Answer from the drawing. Dimensions are ordinates in mm from the lowest x, y and z of the part. Round coordinates to 2 decimals unless told otherwise and drop trailing zeros. Order: outer loops, then holes, each group sorted by start corner. A loop starts at its lowest first (then second) coordinate and runs counter-clockwise, first axis right, second up. Notation, with made-up numbers: M 76.5,34 L 108.5,34 A14 cw 108.5,55 Z; hole C 74.25,51.25 d4. An arc over 180 degrees is marked long. Answer as a JSON object with one key per item and string values. Group by question number.
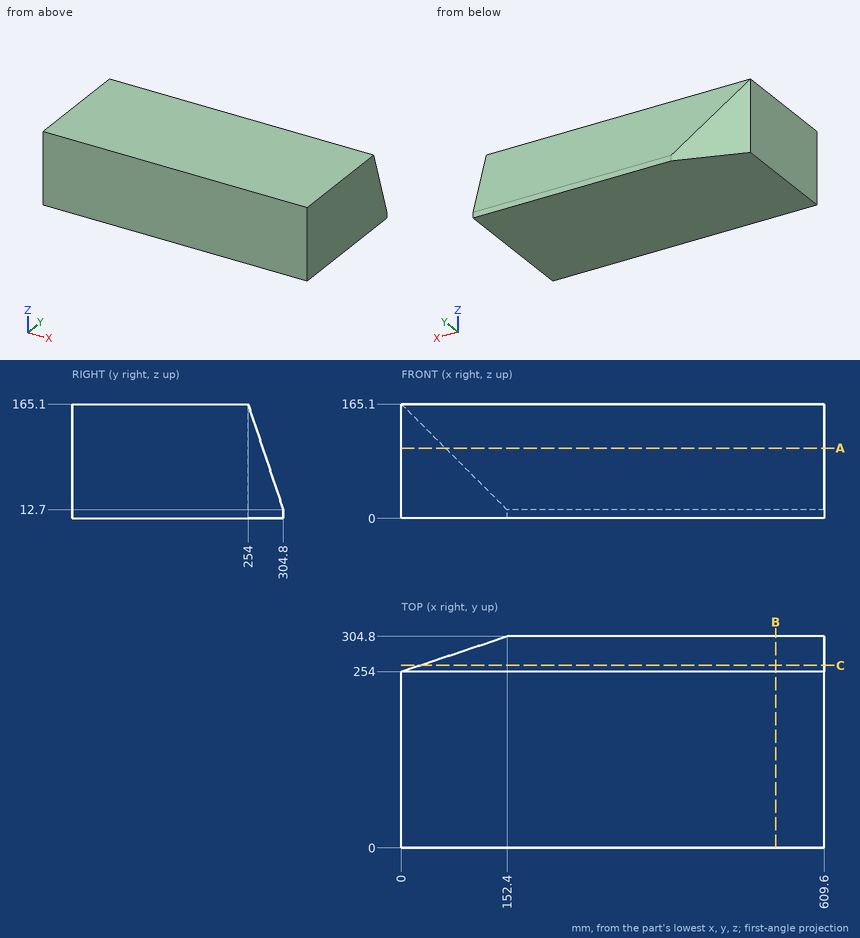
Item 1: Find section C-C (y = 263). Give the vertices of the cut face in (x, z).
Item 2: Consider L1, parallel to Y at x = 351, z = 70; L2, parallel to Y at x = 98, z = 33. Determine where each line is inside the solid, lowest interval first.
Item 3: Find section B-B (x = 540). Give the vertices of the cut face in (y, z).
Item 4: Each of these flat-tipped pins is pushed along its axis until it touches: pin 1 (10 mm diameter, centred on x = 400, z = 77.5, fed in from +Y); pin 2 (10 mm diameter, centred on x = 273.5, z = 90.5, fed in from +Y); pin 3 (3 mm diameter, centred on x = 142, y = 211, fed in from -Z). Where does it stop, or does it pass through?
Item 5: Find section A-A (z = 101.5). Give the vertices of the cut face in (x, y).
Responses:
{
 "1": {"outline": "M 27,0 L 609.6,0 L 609.6,138.1 L 27,138.1 Z"},
 "2": {"L1": "y = 0 to 285.7", "L2": "y = 0 to 286.67"},
 "3": {"outline": "M 0,0 L 304.8,0 L 304.8,12.7 L 254,165.1 L 0,165.1 Z"},
 "4": {"pin 1": "stops at y = 284.87", "pin 2": "stops at y = 280.53", "pin 3": "stops at z = 0"},
 "5": {"outline": "M 0,0 L 609.6,0 L 609.6,275.2 L 63.6,275.2 L 0,254 Z"}
}
